Work out the finished part from the listing and answer in its coordinate system (mm). Face numbers are marked on the shaded views. Coordinates: 2 decimals unless noted, no trailing zeros. Order: outer loops, then holes, each group sorted by start corner. A loop starts at its lowest first (then second) coordinate and runs counter-clockwise, first axis right, second up. Notation, with made-up numbers: M 28.5,49.25 L 47.5,49.25 A19 ccw 47.5,77.25 Z; hole C 88,13 d9. An arc over 180 degrees is marked long. Answer in a Markdown table with one row per item. Add a question column.
Item 1: Flat-ended cylindrical pins translate along their axes: pin 1 Ø9 at (x, y) = (-18.85, -7.5) entering from -Z; pin 2 Ø6 at (x, y) = (18.85, -7.5) entering from -Z. Find the tip coordinate at first contact, or state that the pin passes through.
Item 2: The part is cut by section B-B (z = -35). Write down the section's boundary in (x, y).
Item 3: The part is cut by section A-A (x = 0). Write down the section's boundary in (y, z), then the cut area to 4 significant figures.
Item 4: The part is cut by section D-D (z = 20). Write down the section's boundary in (x, y), then the cut area to 3 significant figures.
Item 5: The mould has two halves that part along Z. Classify the marked faces 1, 2 and 3: released by +Z, released by -Z, zero draft, split by the parting line, or undercut.
Item 6: Consider line 1 (X direction, y = -6.25, z = -19.5); line 2 (Z direction, x = 0, y = -11.25); line 3 (Z direction, x = 21, y = -6.25). Determine where each line is inside the solid, lowest interval first. Write a range as from..to.
Item 7: The part is cut by section C-C (y = -12.25). Write down the section's boundary in (x, z).
from build123d import *

# Parameters (mm, degrees)
F0_R     = 1.5
F0_R_2   = 4.5
F1_DEPTH = 15
F3_D     = 6.8
F3_DEPTH = 20
F3_TIP   = 2.0429261047
F5_D     = 6.8
F5_DEPTH = 20
F5_TIP   = 2.0429261047
F6_SIZE  = 1


with BuildPart() as f1:
    # F0 (on Front) → F1 (new body)
    with BuildSketch(Plane.XZ):
        with BuildLine():
            Line((25, 40), (-25, 40))
            Line((-25, 40), (-25, -40))
            Line((-25, -40), (-12.7, -40))
            ThreePointArc((-12.7, -40), (0, -27.3), (12.7, -40))
            Line((12.7, -40), (25, -40))
            Line((25, -40), (25, 40))
        make_face()
        with Locations((20, -15)):
            Circle(F0_R, mode=Mode.SUBTRACT)
        with Locations((0, 20)):
            Circle(F0_R_2, mode=Mode.SUBTRACT)
    extrude(amount=F1_DEPTH)

    # F3
    with Locations(Plane(origin=(0, 0, -40), x_dir=(1, 0, 0), z_dir=(0, 0, -1))):
        with Locations((-18.85, 7.5)):
            Hole(F3_D / 2, depth=F3_DEPTH)
            with Locations((0, 0, -(F3_DEPTH + F3_TIP / 2))):  # 118° drill point
                Cone(0, F3_D / 2, F3_TIP, mode=Mode.SUBTRACT)

    # F5
    with Locations(Plane(origin=(0, 0, -40), x_dir=(1, 0, 0), z_dir=(0, 0, -1))):
        with Locations((18.85, 7.5)):
            Hole(F5_D / 2, depth=F5_DEPTH)
            with Locations((0, 0, -(F5_DEPTH + F5_TIP / 2))):  # 118° drill point
                Cone(0, F5_D / 2, F5_TIP, mode=Mode.SUBTRACT)

    # F6
    f6_edges = [f1.edges().sort_by_distance(p)[0] for p in [
        (25, -7.5, -40),
        (25, -7.5, 40),
        (25, 0, 0),
        (25, -15, 0),
        (-25, -7.5, 40),
        (0, 0, 40),
        (0, -15, 40),
        (-25, -7.5, -40),
        (-25, 0, 0),
        (-25, -15, 0),
    ]]
    chamfer(f6_edges, length=F6_SIZE)


solid = f1.part
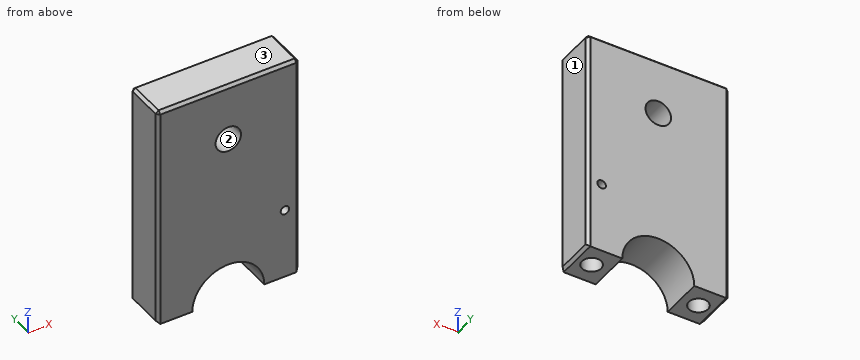
Reply:
| question | item | result |
|---|---|---|
| 1 | pin 1 | stops at z = -40 |
| 1 | pin 2 | stops at z = -19.76 |
| 2 | outline | M -25,-14 L -24,-15 L -11.67,-15 L -11.67,0 L -24,0 L -25,-1 Z; M 11.67,-15 L 24,-15 L 25,-14 L 25,-1 L 24,0 L 11.67,0 Z; hole C -18.85,-7.5 d6.8; hole C 18.85,-7.5 d6.8 |
| 3 | outline | M -15,-27.3 L 0,-27.3 L 0,15.5 L -15,15.5 Z; M -15,24.5 L 0,24.5 L 0,39 L -1,40 L -14,40 L -15,39 Z |
| 3 | area | 873.5 mm2 |
| 4 | outline | M -25,-14 L -24,-15 L -4.5,-15 L -4.5,0 L -24,0 L -25,-1 Z; M 4.5,-15 L 24,-15 L 25,-14 L 25,-1 L 24,0 L 4.5,0 Z |
| 4 | area | 613 mm2 |
| 5 | face 1 | zero draft |
| 5 | face 2 | undercut |
| 5 | face 3 | released by +Z |
| 6 | line 1 | x = -25..-21.09, -16.61..16.61, 21.09..25 |
| 6 | line 2 | z = -27.3..15.5, 24.5..40 |
| 6 | line 3 | z = -19.45..-16.12, -13.88..40 |
| 7 | outline | M -25,-39 L -24,-40 L -12.7,-40 A12.7 cw 12.7,-40 L 24,-40 L 25,-39 L 25,39 L 24,40 L -24,40 L -25,39 Z; hole C 0,20 d9; hole C 20,-15 d3 |
